```python
from build123d import *

# Parameters (mm, degrees)
F0_R         = 18
F1_DEPTH     = 15
F3_DEPTH     = 25
F4_R         = 3
F5_DEPTH     = 25
F4_R_2       = 5
F6_DEPTH     = 2
F7_R         = 3
F8_DEPTH     = 25
F7_R_2       = 5
F9_DEPTH     = 2
F10_R        = 3
F11_DEPTH    = 25
F10_R_2      = 5
F12_DEPTH    = 2
F13_T1_DEPTH = 15
F13_T3_DEPTH = 25


# Not quite as in the source:
# - a fillet or chamfer that OpenCascade refuses, or shapes differently, is made with other operations: its cross-section is extruded or revolved along the edge and cut away or added


with BuildPart() as f1:
    # F0 (on Front) → F1 (new body)
    with BuildSketch(Plane.XZ):
        with BuildLine():
            Line((23, -20.5), (10.4283268073, -20.5))
            ThreePointArc((10.4283268073, -20.5), (0, -23), (-10.4283268073, -20.5))
            Line((-10.4283268073, -20.5), (-23, -20.5))
            Line((-23, -20.5), (-40, -20.5))
            Line((-40, -20.5), (-40, -25.5))
            Line((-40, -25.5), (40, -25.5))
            Line((40, -25.5), (40, -20.5))
            Line((40, -20.5), (23, -20.5))
        make_face()
        with BuildLine():
            Line((-23, -20.5), (-10.4283268073, -20.5))
            ThreePointArc((-10.4283268073, -20.5), (-19.606778376, -12.0239029319), (-23, 0))
            Line((-23, 0), (-23, -20.5))
        make_face()
        with BuildLine():
            ThreePointArc((10.4283268073, -20.5), (19.606778376, -12.0239029319), (23, 0))
            ThreePointArc((23, 0), (18.2619823677, 13.9821314541), (6, 22.2036033112))
            Line((6, 22.2036033112), (6, 19.0559069812))
            Line((6, 19.0559069812), (-6, 19.0559069812))
            Line((-6, 19.0559069812), (-6, 22.2036033112))
            ThreePointArc((-6, 22.2036033112), (-18.2619823677, 13.9821314541), (-23, 0))
            ThreePointArc((-23, 0), (-19.606778376, -12.0239029319), (-10.4283268073, -20.5))
            Line((-10.4283268073, -20.5), (10.4283268073, -20.5))
        make_face()
        Circle(F0_R, mode=Mode.SUBTRACT)
        with BuildLine():
            Line((23, -20.5), (23, 0))
            ThreePointArc((23, 0), (19.606778376, -12.0239029319), (10.4283268073, -20.5))
            Line((10.4283268073, -20.5), (23, -20.5))
        make_face()
        with BuildLine():
            ThreePointArc((-10.4283268073, -20.5), (0, -23), (10.4283268073, -20.5))
            Line((10.4283268073, -20.5), (-10.4283268073, -20.5))
        make_face()
        with BuildLine():
            ThreePointArc((-6, 22.2036033112), (0, 23), (6, 22.2036033112))
            Line((6, 22.2036033112), (6, 34.0559069812))
            Line((6, 34.0559069812), (-6, 34.0559069812))
            Line((-6, 34.0559069812), (-6, 22.2036033112))
        make_face()
        with BuildLine():
            Line((6, 19.0559069812), (6, 22.2036033112))
            ThreePointArc((6, 22.2036033112), (0, 23), (-6, 22.2036033112))
            Line((-6, 22.2036033112), (-6, 19.0559069812))
            Line((-6, 19.0559069812), (6, 19.0559069812))
        make_face()
    extrude(amount=F1_DEPTH)

    # F2 (on face) → F3 (cut)
    with BuildSketch(Plane.XZ.offset(15)):
        with BuildLine():
            Line((1, 34.0559069812), (-1, 34.0559069812))
            Line((-1, 34.0559069812), (-1, 17.9722007556))
            ThreePointArc((-1, 17.9722007556), (0, 18), (1, 17.9722007556))
            Line((1, 17.9722007556), (1, 34.0559069812))
        make_face()
    extrude(amount=-F3_DEPTH, mode=Mode.SUBTRACT)

    # F4 (on face) → F5 (cut)
    with BuildSketch(Plane.XY.offset(-20.5)):
        with Locations((31.5, -7.5)):
            Circle(F4_R)
    extrude(amount=-F5_DEPTH, mode=Mode.SUBTRACT)

    # F4 (on face) → F6 (cut)
    with BuildSketch(Plane.XY.offset(-20.5)):
        with Locations((31.5, -7.5)):
            Circle(F4_R_2)
        with Locations((31.5, -7.5)):
            Circle(F4_R, mode=Mode.SUBTRACT)
    extrude(amount=-F6_DEPTH, mode=Mode.SUBTRACT)

    # F7 (on face) → F8 (cut)
    with BuildSketch(Plane.XY.offset(-20.5)):
        with Locations((-31.5, -7.5)):
            Circle(F7_R)
    extrude(amount=-F8_DEPTH, mode=Mode.SUBTRACT)

    # F7 (on face) → F9 (cut)
    with BuildSketch(Plane.XY.offset(-20.5)):
        with Locations((-31.5, -7.5)):
            Circle(F7_R_2)
        with Locations((-31.5, -7.5)):
            Circle(F7_R, mode=Mode.SUBTRACT)
    extrude(amount=-F9_DEPTH, mode=Mode.SUBTRACT)

    # F10 (on face) → F11 (cut)
    with BuildSketch(Plane.YZ.offset(6)):
        with Locations((-7.5, 28.1297551462)):
            Circle(F10_R)
    extrude(amount=-F11_DEPTH, mode=Mode.SUBTRACT)

    # F10 (on face) → F12 (cut)
    with BuildSketch(Plane.YZ.offset(6)):
        with Locations((-7.5, 28.1297551462)):
            Circle(F10_R_2)
        with Locations((-7.5, 28.1297551462)):
            Circle(F10_R, mode=Mode.SUBTRACT)
    extrude(amount=-F12_DEPTH, mode=Mode.SUBTRACT)

    # F13: fillet of radius 2 on 6 edges, made by hand

    # F13_s2 → F13_t1 (join)
    with BuildSketch(Plane.XZ):
        with BuildLine():
            ThreePointArc((25, -20.5), (23.5857864376, -19.9142135624), (23, -18.5))
            Line((23, -18.5), (23, -20.5))
            Line((23, -20.5), (25, -20.5))
        make_face()
        with BuildLine():
            ThreePointArc((-25, -20.5), (-23.5857864376, -19.9142135624), (-23, -18.5))
            Line((-23, -18.5), (-23, -20.5))
            Line((-23, -20.5), (-25, -20.5))
        make_face()
    extrude(amount=F13_T1_DEPTH)

    # F13_s4 → F13_t3 (cut)
    with BuildSketch(Plane.XZ.offset(-5)):
        with BuildLine():
            ThreePointArc((-6, 32.0559069812), (-5.4142135624, 33.4701205436), (-4, 34.0559069812))
            Line((-4, 34.0559069812), (-6, 34.0559069812))
            Line((-6, 34.0559069812), (-6, 32.0559069812))
        make_face()
        with BuildLine():
            ThreePointArc((4, 34.0559069812), (5.4142135624, 33.4701205436), (6, 32.0559069812))
            Line((6, 32.0559069812), (6, 34.0559069812))
            Line((6, 34.0559069812), (4, 34.0559069812))
        make_face()
        with BuildLine():
            ThreePointArc((38, -20.5), (39.4142135624, -21.0857864376), (40, -22.5))
            Line((40, -22.5), (40, -20.5))
            Line((40, -20.5), (38, -20.5))
        make_face()
        with BuildLine():
            ThreePointArc((-40, -22.5), (-39.4142135624, -21.0857864376), (-38, -20.5))
            Line((-38, -20.5), (-40, -20.5))
            Line((-40, -20.5), (-40, -22.5))
        make_face()
    extrude(amount=F13_T3_DEPTH, mode=Mode.SUBTRACT)


solid = f1.part
```
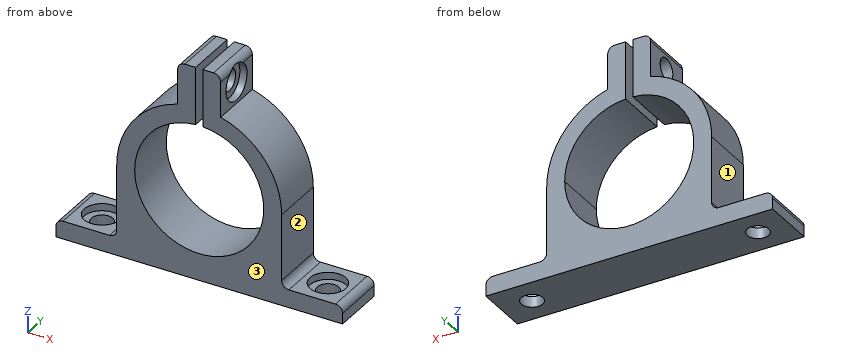
Part model, mm, in its own coordinate system. Face numbers are marked on the shaded views. A direction names the side the tool comes from. Coordinates: 2 decimals unless noted, no trailing zeros. Write each loop counter-clockwise with the first axis right and the second up, starting at its lowest first coordinate (ties: lowest second). Pieces come first, ordered by that corner, then holes.
Item 1: Slice it at D-D (x = 30.5). Write the cut outline in (y, z), and give its area (3 significant figures).
Item 2: Which spindle directions (+Z, -Z, +X, -X, +Y, -Y) get a long thin tool onto all of the face, cutting with end or side? Do the marked faces 1, 2 and 3. Say none if no direction does.
Item 3: Slice it at A-A (x = 2.5). Write the cut outline in (y, z).
Item 4: Probe line 1 (Z direction, x = -2.6, y = -7.5); line 2 (X direction, y = -9.25, z = 25); line 3 (Z direction, x = 25.5, y = -3.5). List the from-to ranges inside material, lowest first.
Item 5: Pin check, flat tips, straight feed: pin 1 (7 mm diameter, centred on x = -31.5, y = -7.5, fed in from +Z); pin 2 (8 mm diameter, centred on y = -7.5, z = 28.13, fed in from +X); pin 3 (3 mm diameter, centred on y = -6, z = 27.5, fed in from -X); pin 4 (5 mm diameter, centred on y = -7.5, z = 28.13, fed in from -X). Stop position of each tip, or through.
Item 6: Slice it at B-B (z = 15). Write the cut outline in (x, y).
Results found:
1. outline: (-15, -25.5) - (-10.33, -25.5) - (-10.33, -22.5) - (-12.4, -22.5) - (-12.4, -20.5) - (-15, -20.5) - close; (-4.67, -25.5) - (0, -25.5) - (0, -20.5) - (-2.6, -20.5) - (-2.6, -22.5) - (-4.67, -22.5) - close
1. area: 38.4 mm2
2. face 1: +Z, -X, +Y, -Y
2. face 2: +Z, +X, +Y, -Y
2. face 3: +Z, -Z, +X, -X, -Y
3. outline: (-15, -25.5) - (0, -25.5) - (0, -17.83) - (-15, -17.83) - close; (-15, 17.83) - (0, 17.83) - (0, 34.06) - (-15, 34.06) - close; hole circle Ø6 at (-7.5, 28.13)
4. line 1: z = -25.5 to -17.81, 17.81 to 25.13, 31.13 to 34.06
4. line 2: x = -6 to -1, 1 to 4
4. line 3: z = -25.5 to -20.5
5. pin 1: stops at z = -22.5
5. pin 2: stops at x = 4
5. pin 3: stops at x = -6
5. pin 4: passes through
6. outline: (-17.44, -15) - (-9.95, -15) - (-9.95, 0) - (-17.44, 0) - close; (9.95, -15) - (17.44, -15) - (17.44, 0) - (9.95, 0) - close
